Could you check a few things on this model? Use its own coordinates, in mm. A direction names the side the tool comes from. Round coordinates to 2 decimals unless told otherwise and drop trailing zeros. Loops run counter-clockwise (first coordinate to the right, second up) from the corner with the lowest first, then second, coordinate; pieces in that order, holes last. Notation, with made-up numbers: (-1, -5) -> (30, -5) arc R23 cw to (30, 5) -> close; hole circle Ø4 at (-10, 0). An arc over 180 degrees is marked (long way). One line per item, written item: value.
Autodesk Inventor part; units mm, degrees
ref_plane "YZ Plane" through (0, 0, 0) normal (1, 0, 0) x (0, 1, 0)
ref_plane "XZ Plane" through (0, 0, 0) normal (0, 1, 0) x (-1, 0, 0)
ref_plane "XY Plane" through (0, 0, 0) normal (0, 0, 1) x (1, 0, 0)
sketch "Boceto1" plane through (0, 0, 0) normal (0, 1, 0) x (-1, 0, 0)
  circle A0 centre (16.5, 0) radius 1.5
  circle A1 centre (0, -16.5) radius 1.5
  circle A2 centre (-16.5, 0) radius 1.5
  circle A3 centre (0, 16.5) radius 1.5
  line L0 (3.5, 11) -> (3.5, 16.5)
  line L1 (3.5, -16.5) -> (3.5, -11)
  line L2 (11, -3.5) -> (16.5, -3.5)
  line L3 (-16.5, -3.5) -> (-11, -3.5)
  arc A4 (3.5, 16.5) -> (-3.5, 16.5) centre (0, 16.5) ccw
  arc A5 (16.5, -3.5) -> (16.5, 3.5) centre (16.5, 0) ccw
  arc A6 (-3.5, -16.5) -> (3.5, -16.5) centre (0, -16.5) ccw
  arc A7 (-16.5, 3.5) -> (-16.5, -3.5) centre (-16.5, 0) ccw
  line L4 (16.5, 3.5) -> (11, 3.5)
  line L5 (-11, 3.5) -> (-16.5, 3.5)
  line L6 (-3.5, 16.5) -> (-3.5, 11)
  line L7 (-3.5, -11) -> (-3.5, -16.5)
  arc A8 (11, -3.5) -> (3.5, -11) centre (11, -11) ccw
  arc A9 (-3.5, -11) -> (-11, -3.5) centre (-11, -11) ccw
  arc A10 (-11, 3.5) -> (-3.5, 11) centre (-11, 11) ccw
  arc A11 (3.5, 11) -> (11, 3.5) centre (11, 11) ccw
  circle A12 centre (0, 0) radius 5
  dimension "d12" = 7.5
  dimension "d15" = 10
extrude "Extrusión1" add sketch "Boceto1" along normal blind 2
properties part number "Base Motor"
(1) If I drill on L1, parallel to Z at x = 0, y = 1.2; L2, parallel to Z at x = -16.5, y = 1.05; L3, parallel to X at y = 1.05, z = -12, over which ranges is the centre line in solid material (lowest first)?
Recorded:
L1: -20 to -18, -15 to -5, 5 to 15, 18 to 20
L2: -3.5 to -1.5, 1.5 to 3.5
L3: -3.5 to 3.5
(2) Thinking about a two-plate mould opening in Z: for faces 4 (the face through (-14, 1, 3.5)), 5 (the face through (20, 1, 0)), 6 (the face through (0, 1, 18)), 7 (the face through (1.08, 0.99, 4.88)), which applies, released by +Z, released by -Z, zero draft, split by the parting line, or undercut?
Recorded:
face 4: released by +Z
face 5: split by the parting line
face 6: undercut
face 7: undercut
(3) If we section it at C-C, the plane y = 0.85: Please give me the cut outline in (x, z), then the cut area to 3 significant figures.
Recorded:
outline: (-16.5, -3.5) -> (-11, -3.5) arc R7.5 cw to (-3.5, -11) -> (-3.5, -16.5) arc R3.5 ccw to (3.5, -16.5) -> (3.5, -11) arc R7.5 cw to (11, -3.5) -> (16.5, -3.5) arc R3.5 ccw to (16.5, 3.5) -> (11, 3.5) arc R7.5 cw to (3.5, 11) -> (3.5, 16.5) arc R3.5 ccw to (-3.5, 16.5) -> (-3.5, 11) arc R7.5 cw to (-11, 3.5) -> (-16.5, 3.5) arc R3.5 ccw to start; hole circle Ø3 at (-16.5, 0); hole circle Ø10 at (0, 0); hole circle Ø3 at (0, -16.5); hole circle Ø3 at (0, 16.5); hole circle Ø3 at (16.5, 0)
area: 431 mm²
(4) If we section it at D-D, the plane z = -16: Please give me the cut outline in (x, y).
Recorded:
outline: (-3.5, 0) -> (-1.41, 0) -> (-1.41, 2) -> (-3.5, 2) -> close; (1.41, 0) -> (3.5, 0) -> (3.5, 2) -> (1.41, 2) -> close
(5) I'm going to push flat-ended pins straight in: pin 1 Ø2.5 at (x, z) = (16.5, 0) entering from +Y; pin 2 Ø1 at (x, y) = (-13.5, 1.5) entering from -Z; pin 3 Ø1 at (y, z) = (1, 13) entering from -X; pin 4 Ø0.6 at (x, y) = (13, 1.5) entering from +Z. Where does each tip first touch, or does it pass through?
Recorded:
pin 1: through
pin 2: z = -3.5
pin 3: x = -3.5
pin 4: z = 3.5
(6) For faces 1 (the face through (-3.5, 1, 14)), 2 (the face through (3.5, 1, -14)), 3 (the face through (3.5, 1, 14)), which set-ups out of +Z, -Z, +X, -X, +Y, -Y let a thin tool reach every point of the face, with its end or its side?
Recorded:
face 1: +Z, -X, +Y, -Y
face 2: -Z, +X, +Y, -Y
face 3: +Z, +X, +Y, -Y
(7) If we section it at B-B, the plane x = 0: Please give me the cut outline in (y, z), then the cut area to 3 significant figures.
Recorded:
outline: (0, -20) -> (2, -20) -> (2, -18) -> (0, -18) -> close; (0, -15) -> (2, -15) -> (2, -5) -> (0, -5) -> close; (0, 5) -> (2, 5) -> (2, 15) -> (0, 15) -> close; (0, 18) -> (2, 18) -> (2, 20) -> (0, 20) -> close
area: 48.0 mm²
(8) If we section it at A-A, the plane z = 0: Please give me the cut outline in (x, y).
Recorded:
outline: (-20, 0) -> (-18, 0) -> (-18, 2) -> (-20, 2) -> close; (-15, 0) -> (-5, 0) -> (-5, 2) -> (-15, 2) -> close; (5, 0) -> (15, 0) -> (15, 2) -> (5, 2) -> close; (18, 0) -> (20, 0) -> (20, 2) -> (18, 2) -> close
